Part model, mm, in its own coordinate system. A direction names the side the tool comes from. Round coordinates to 2 decimals unless told otherwise and drop trailing zeros. Loops run counter-clockwise (first coordinate to the right, second up) from the corner with the lowest first, then second, coordinate; pieces in that order, holes last.
from build123d import *

# Parameters (mm, degrees)
F0_W     = 29
F0_H     = 29
F1_DEPTH = 5
F0_W_2   = 24
F0_H_2   = 24
F2_DEPTH = 4


with BuildPart() as f1:
    # F0 (on Top) → F1 (new body)
    with BuildSketch(Plane.XY):
        with Locations((14, 14)):
            Rectangle(F0_W, F0_H)
        with BuildLine():
            Line((0.5, 27.5), (11.566837, 27.5))
            ThreePointArc((11.566837, 27.5), (13.5, 26.01284), (15.433163, 27.5))
            Line((15.433163, 27.5), (27.5, 27.5))
            Line((27.5, 27.5), (27.5, 0.5))
            Line((27.5, 0.5), (0.5, 0.5))
            Line((0.5, 0.5), (0.5, 27.5))
        make_face(mode=Mode.SUBTRACT)
    extrude(amount=F1_DEPTH)

    # F0 (on Top) → F2 (join)
    with BuildSketch(Plane.XY):
        with BuildLine():
            ThreePointArc((15.433163, 27.5), (13.5, 26.01284), (11.566837, 27.5))
            Line((11.566837, 27.5), (0.5, 27.5))
            Line((0.5, 27.5), (0.5, 0.5))
            Line((0.5, 0.5), (27.5, 0.5))
            Line((27.5, 0.5), (27.5, 27.5))
            Line((27.5, 27.5), (15.433163, 27.5))
        make_face()
        with Locations((14, 14)):
            Rectangle(F0_W_2, F0_H_2, mode=Mode.SUBTRACT)
    extrude(amount=F2_DEPTH)


solid = f1.part
1) Wall check: line 1 along Y through (x, z) = (25.5, 1.4); line 2 along Y through (x, z) = (15.75, 4.5). Give the ranges that are in metal, low to high.
Values:
line 1: y = -0.5 to 2, 26 to 28.5
line 2: y = -0.5 to 0.5, 27.5 to 28.5
2) Drop flat-ended pins along their axis: pin 1 Ø4 at (x, y) = (23.5, 17.5) entering from +Z; pin 2 Ø4 at (x, y) = (19, 3) entering from +Z. Give the stop position or say it passes through.
Values:
pin 1: passes through
pin 2: stops at z = 4
3) Tool access for faces 5 (the face through (14, -0.5, 2)), 6 (the face through (2, 14, 2)), 7 (the face through (27.5, 14.2, 4.5)): list every direction of +Z, -Z, +X, -X, +Y, -Y with a clear straight run to the whole face (end or side of a thin tool).
Values:
face 5: +Z, -Z, +X, -X, -Y
face 6: +Z, -Z
face 7: +Z
4) Mould opens along Y. For faces 1 (the face through (14, 2, 2)), 2 (the face through (14, 28.5, 2)), 3 (the face through (-0.5, 14, 2)), 4 (the face through (0.5, 13.8, 4.5)) say: released by +Y, released by -Y, zero draft, split by the parting line, or undercut.
Values:
face 1: undercut
face 2: released by +Y
face 3: zero draft
face 4: undercut
5) Slice it at A-A, the plane x = 25.25. Give the cut face in (y, z).
Values:
outline: (-0.5, 0) - (2, 0) - (2, 4) - (0.5, 4) - (0.5, 5) - (-0.5, 5) - close; (26, 0) - (28.5, 0) - (28.5, 5) - (27.5, 5) - (27.5, 4) - (26, 4) - close
6) Slice it at B-B, the plane z = 3.6. Give the cut face in (x, y).
Values:
outline: (-0.5, -0.5) - (28.5, -0.5) - (28.5, 28.5) - (-0.5, 28.5) - close; hole (2, 2) - (26, 2) - (26, 26) - (2, 26) - close
7) Slice it at D-D, the plane y = 26.5. Give the cut face in (x, z).
Values:
outline: (-0.5, 0) - (28.5, 0) - (28.5, 5) - (27.5, 5) - (27.5, 4) - (14.81, 4) - (14.81, 5) - (12.19, 5) - (12.19, 4) - (0.5, 4) - (0.5, 5) - (-0.5, 5) - close
